from build123d import *

# Parameters (mm, degrees)
SKETCH1_W           = 63.5
SKETCH1_H           = 40.132
BOSS_EXTRUDE1_DEPTH = 6.35
CUT_EXTRUDE1_DEPTH  = 7.35
SKETCH3_W           = 12.7
SKETCH3_H           = 6.35
SKETCH3_W_2         = 15.875
BOSS_EXTRUDE2_DEPTH = 6.35
SKETCH4_W           = 2.54
SKETCH4_H           = 37.084
BOSS_EXTRUDE7_DEPTH = 6.35
SKETCH6_W           = 2.54
SKETCH6_H           = 46.482
BOSS_EXTRUDE8_DEPTH = 6.35


with BuildPart() as part:
    # Sketch1 → Boss-Extrude1 (new body)
    with BuildSketch(Plane(origin=(0, 0, 0), x_dir=(0, 0, -1), z_dir=(1, 0, 0))):
        Rectangle(SKETCH1_W, SKETCH1_H)
    extrude(amount=BOSS_EXTRUDE1_DEPTH)

    # Sketch2 → Cut-Extrude1 (cut, through all)
    with BuildSketch(Plane.ZY):
        Polygon((-31.75, -20.066), (-31.75, 20.066), (-6.35, 20.066), align=None)
    extrude(amount=-CUT_EXTRUDE1_DEPTH, mode=Mode.SUBTRACT)

    # Sketch3 → Boss-Extrude2 (add, through all)
    with BuildSketch(Plane.ZY):
        with Locations((25.4, 23.241)):
            Rectangle(SKETCH3_W, SKETCH3_H)
        with Locations((0, 23.241)):
            Rectangle(SKETCH3_W, SKETCH3_H)
        with Locations((7.9375, -23.241)):
            Rectangle(SKETCH3_W_2, SKETCH3_H)
        with Locations((-23.8125, -23.241)):
            Rectangle(SKETCH3_W_2, SKETCH3_H)
    extrude(amount=-BOSS_EXTRUDE2_DEPTH)

    # Sketch4 → Boss-Extrude7 (add)
    with BuildSketch(Plane.ZY):
        with Locations((30.48, 2.667)):
            Rectangle(SKETCH4_W, SKETCH4_H)
    extrude(amount=-BOSS_EXTRUDE7_DEPTH)

    # Sketch6 → Boss-Extrude8 (add)
    with BuildSketch(Plane(origin=(6.35, 0, 0), x_dir=(0, 0, -1), z_dir=(1, 0, 0))):
        with Locations((-33.02, 3.175)):
            Rectangle(SKETCH6_W, SKETCH6_H)
    extrude(amount=-BOSS_EXTRUDE8_DEPTH)


solid = part.part
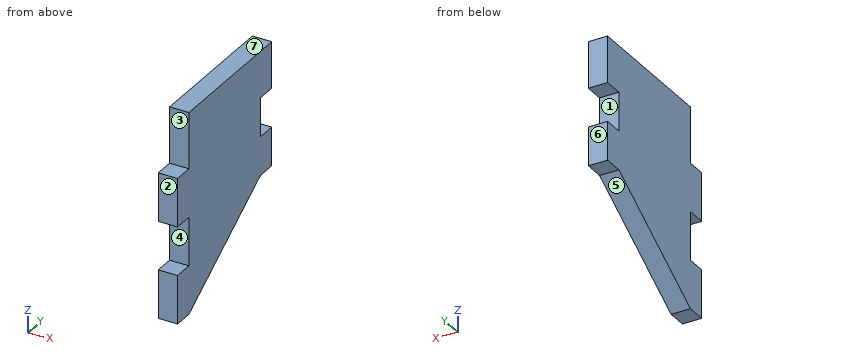
Could you check a few things on this model? Use its own coordinates, in mm. Face numbers are marked on the shaded views. A direction names the side the tool comes from. Round coordinates to 2 decimals unless told otherwise and drop trailing zeros. Write each loop counter-clockwise with the first axis right and the second up, starting at its lowest first coordinate (ties: lowest second). Pieces come first, ordered by that corner, then holes. Notation, with made-up numbers: (50.5, -19.5) - (107.5, -19.5) arc R17 ccw to (107.5, -4.5) - close; hole circle Ø6 at (86.25, 88.5). An arc over 180 degrees is marked (long way). Use a Markdown table: item, result.
Q1. Please list where these lines run through material, in increasing order: L1, parallel to Z at x = 4, y = 20.5; L2, parallel to Y at x = 6, z = 6.5; L3, parallel to Z at x = 2, y = -20.5 (3 decimals).
Output values:
| item | result |
|---|---|
| L1 | -6.35 to 6.35, 19.05 to 34.29 |
| L2 | -26.42 to 20.07 |
| L3 | -31.75 to -15.875, 0 to 15.875 |
Q2. For pin 1 (1.9 mm diameter, centred on x = 2.5, y = -22.5, fed in from +Z) (3 decimals); pin 2 (1.9 mm diameter, centred on x = 2, z = 11, fed in from +Y); pin 3 (1.9 mm diameter, centred on x = 2.5, z = -9.5, fed in from -Y), each with a flat end and sliding along its axis, tell me the tip position at first contact or that it passes through.
Output values:
| item | result |
|---|---|
| pin 1 | z = 15.875 |
| pin 2 | y = 20.07 |
| pin 3 | y = -20.07 |
Q3. I want a section at B-B (z = 14). List the corners of the cut face in (x, y) for me, plus the area to 3 significant figures.
Output values:
| item | result |
|---|---|
| outline | (0, -26.42) - (6.35, -26.42) - (6.35, 20.07) - (0, 20.07) - close |
| area | 295 mm2 |
Q4. For the marked faces 1, 2 and 3, which set-ups out of +Z, -Z, +X, -X, +Y, -Y let a thin tool reach every point of the face, with its end or its side?
Output values:
| item | result |
|---|---|
| face 1 | +X, -X, +Y |
| face 2 | +Z, -Z, +X, -X, -Y |
| face 3 | +Z, +X, -X, -Y |
Q5. Thinking about a two-plate mould opening in Z: for the marked faces 4, 5, 6 and 7, which applies, released by +Z, released by -Z, zero draft, split by the parting line, or undercut?
Output values:
| item | result |
|---|---|
| face 4 | undercut |
| face 5 | released by -Z |
| face 6 | zero draft |
| face 7 | released by +Z |
Q6. I want a section at C-C (y = 15.5). List the corners of the cut face in (x, z) for me, plus the area to 3 significant figures.
Output values:
| item | result |
|---|---|
| outline | (0, -9.24) - (6.35, -9.24) - (6.35, 34.29) - (0, 34.29) - close |
| area | 276 mm2 |
Q7. I want a section at A-A (x = 5.5). List the corners of the cut face in (y, z) for me (3 decimals).
Output values:
| item | result |
|---|---|
| outline | (-26.416, -31.75) - (-20.066, -31.75) - (20.066, -6.35) - (26.416, -6.35) - (26.416, 6.35) - (20.066, 6.35) - (20.066, 19.05) - (26.416, 19.05) - (26.416, 34.29) - (-20.066, 34.29) - (-20.066, 15.875) - (-26.416, 15.875) - (-26.416, 0) - (-20.066, 0) - (-20.066, -15.875) - (-26.416, -15.875) - close |
